The listing builds one solid part. Answer for the finished solid, in the listing's coordinates (mm). Coordinates: 2 decimals unless noted, no trailing zeros. Order: outer loops, then holes, each group sorted by start corner. A loop starts at its lowest first (then second) coordinate and runs counter-clockwise, first axis right, second up.
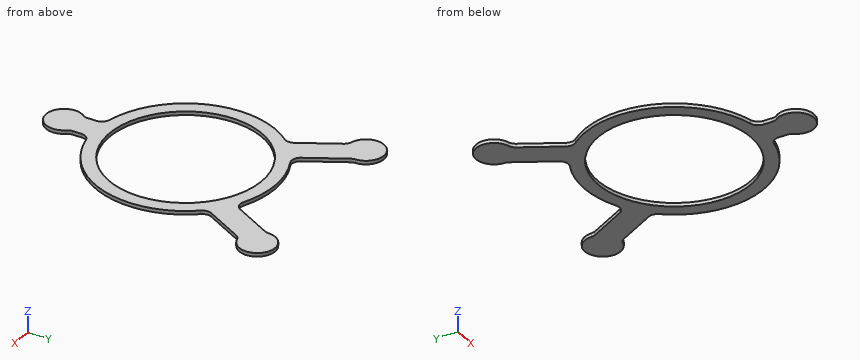
```python
from build123d import *

# Parameters (mm, degrees)
SKETCH1_R          = 53.975
BASE_EXTRUDE_DEPTH = 2.54


with BuildPart() as part:
    # Sketch1 → Base-Extrude (new body)
    with BuildSketch(Plane.XY):
        with BuildLine():
            Line((50.008687045, 171.923839684), (35.512218796, 145.748360325))
            ThreePointArc((35.512218796, 145.748360325), (31.899714725, 142.779219777), (27.233844451, 143.088470227))
            ThreePointArc((27.233844451, 143.088470227), (0, 149.225), (-27.233844451, 143.088470227))
            ThreePointArc((-27.233844451, 143.088470227), (-31.899714725, 142.779219777), (-35.512218796, 145.748360325))
            Line((-35.512218796, 145.748360325), (-50.008687045, 171.923839684))
            ThreePointArc((-50.008687045, 171.923839684), (-50.585784013, 173.351051132), (-50.802464763, 174.875197739))
            ThreePointArc((-50.802464763, 174.875197739), (-71.318679333, 184.632909546), (-66.815120037, 162.365310806))
            ThreePointArc((-66.815120037, 162.365310806), (-64.556557847, 161.234114711), (-62.917690155, 159.311923133))
            Line((-62.917690155, 159.311923133), (-48.421221906, 133.136443774))
            ThreePointArc((-48.421221906, 133.136443774), (-47.652448943, 129.483338569), (-49.069283461, 126.0295335))
            ThreePointArc((-49.069283461, 126.0295335), (-60.040658228, 65.052086332), (-13.854545455, 23.754833224))
            ThreePointArc((-13.854545455, 23.754833224), (-10.284188444, 21.528009466), (-8.89, 17.557816546))
            Line((-8.89, 17.557816546), (-8.89, 11.43))
            ThreePointArc((-8.89, 11.43), (-9.215861057, 9.421953686), (-10.16, 7.62))
            ThreePointArc((-10.16, 7.62), (0, -12.7), (10.16, 7.62))
            ThreePointArc((10.16, 7.62), (9.215861057, 9.421953686), (8.89, 11.43))
            Line((8.89, 11.43), (8.89, 17.557816546))
            ThreePointArc((8.89, 17.557816546), (10.284188444, 21.528009466), (13.854545455, 23.754833224))
            ThreePointArc((13.854545455, 23.754833224), (60.040658228, 65.052086332), (49.069283461, 126.0295335))
            ThreePointArc((49.069283461, 126.0295335), (47.652448943, 129.483338569), (48.421221906, 133.136443774))
            Line((48.421221906, 133.136443774), (62.917690155, 159.311923133))
            ThreePointArc((62.917690155, 159.311923133), (64.556557847, 161.234114711), (66.815120037, 162.365310806))
            ThreePointArc((66.815120037, 162.365310806), (71.318679333, 184.632909546), (50.802464763, 174.875197739))
            ThreePointArc((50.802464763, 174.875197739), (50.585784013, 173.351051132), (50.008687045, 171.923839684))
        make_face()
        with Locations((0, 85.725)):
            Circle(SKETCH1_R, mode=Mode.SUBTRACT)
    extrude(amount=BASE_EXTRUDE_DEPTH)


solid = part.part
```
(1) Find section C-C (z = 2.15). Write down the section's boundary in (x, y) (3 decimals), and give its area (3 significant figures).
(2) Consider line 1 (X direction, y = 163, z = 1.65); line 2 (X direction, y = 86, z = 1.1); line 3 (Y direction, x = -18.5, z = 0.9). Determine where each line is inside the solid, lowest interval first.
(3) Find section B-B (y = 76.5). Write down the section's boundary in (x, z), and give its area (3 significant figures).
(4) Find section D-D (y = 0). Write down the section's boundary in (x, z), and give its area (3 significant figures).
(5) Each of these flat-tipped pins is pushed along its axis until it touches: pin 1 Ø0.8 at (y, z) = (15.5, 1) entering from +X; pin 2 Ø1.3 at (y, z) = (14.5, 1) entering from -X. Where does it stop, or does it pass through?
(6) Find section A-A (x = 0). Write down the section's boundary in (y, z) (3 decimals).
Findings below:
1. outline: (-66.815, 162.365) arc R6.35 cw to (-62.918, 159.312) - (-48.421, 133.136) arc R6.35 cw to (-49.069, 126.03) arc R63.5 ccw to (-13.855, 23.755) arc R6.35 cw to (-8.89, 17.558) - (-8.89, 11.43) arc R6.35 cw to (-10.16, 7.62) arc R12.7 ccw (long way) to (10.16, 7.62) arc R6.35 cw to (8.89, 11.43) - (8.89, 17.558) arc R6.35 cw to (13.855, 23.755) arc R63.5 ccw to (49.069, 126.03) arc R6.35 cw to (48.421, 133.136) - (62.918, 159.312) arc R6.35 cw to (66.815, 162.365) arc R12.7 ccw (long way) to (50.802, 174.875) arc R6.35 cw to (50.009, 171.924) - (35.512, 145.748) arc R6.35 cw to (27.234, 143.088) arc R63.5 ccw to (-27.234, 143.088) arc R6.35 cw to (-35.512, 145.748) - (-50.009, 171.924) arc R6.35 cw to (-50.802, 174.875) arc R12.7 ccw (long way) to start; hole circle Ø107.95 at (0, 85.725)
1. area: 6,470 mm2
2. line 1: x = -68.61 to -45.07, 45.07 to 68.61
2. line 2: x = -63.5 to -53.97, 53.97 to 63.5
2. line 3: y = 24.98 to 35.02, 136.43 to 146.47
3. outline: (-62.83, 0) - (-53.18, 0) - (-53.18, 2.54) - (-62.83, 2.54) - close; (53.18, 0) - (62.83, 0) - (62.83, 2.54) - (53.18, 2.54) - close
3. area: 49.0 mm2
4. outline: (-12.7, 0) - (12.7, 0) - (12.7, 2.54) - (-12.7, 2.54) - close
4. area: 64.5 mm2
5. pin 1: stops at x = 8.89
5. pin 2: stops at x = -8.89
6. outline: (-12.7, 0) - (31.75, 0) - (31.75, 2.54) - (-12.7, 2.54) - close; (139.7, 0) - (149.225, 0) - (149.225, 2.54) - (139.7, 2.54) - close
